Verification items for the finished model (mm, model axes). A direction names the side the tool comes from. Give positions to 0.01 mm unless a question says otherwise; leave off trailing zeros. Write each loop counter-clockwise with the first axis right and the second up, starting at its lowest first coordinate (ties: lowest second). Pieces come first, ordered by that corner, then holes. Notation, with made-up numbers: (17, 39.25) -> (49, 39.25) arc R14 cw to (49, 43.25) -> close; hole circle Ø10 at (-25.75, 89). An arc over 180 degrees is marked (long way). Answer as CSV lines item,"result".
```python
from build123d import *

# Parameters (mm, degrees)
F0_W     = 127
F0_H     = 73.025
F1_DEPTH = 22.225
F2_W     = 47.625
F2_H     = 22.225
F3_DEPTH = 6.35
F4_R     = 9.525
F5_DEPTH = 41.275


with BuildPart() as f1:
    # F0 (on Front) → F1 (new body)
    with BuildSketch(Plane.XZ):
        with Locations((0.306161, -6.260679)):
            Rectangle(F0_W, F0_H)
    extrude(amount=F1_DEPTH)

    # F2 (on face) → F3 (join)
    with BuildSketch(Plane.XY.offset(30.251821)):
        with Locations((39.993661, -11.1125)):
            Rectangle(F2_W, F2_H)
        with Locations((-39.381339, -11.1125)):
            Rectangle(F2_W, F2_H)
    extrude(amount=F3_DEPTH)

    # F4 (on face) → F5 (cut)
    with BuildSketch(Plane.XY.offset(36.601821)):
        with Locations((-34.618839, -11.1125)):
            Circle(F4_R)
        with Locations((41.581161, -11.1125)):
            Circle(F4_R)
    extrude(amount=-F5_DEPTH, mode=Mode.SUBTRACT)


solid = f1.part
```
1) Section check A-A (y = -14.5). Record the boundary of the cut face in (x, z).
Reported:
outline,"(-63.19, -42.77) -> (63.81, -42.77) -> (63.81, 36.6) -> (50.48, 36.6) -> (50.48, -4.67) -> (32.68, -4.67) -> (32.68, 36.6) -> (16.18, 36.6) -> (16.18, 30.25) -> (-15.57, 30.25) -> (-15.57, 36.6) -> (-25.72, 36.6) -> (-25.72, -4.67) -> (-43.52, -4.67) -> (-43.52, 36.6) -> (-63.19, 36.6) -> close"
2) Section check C-C (z = 0). State how many separate pieces and enclosed holes the cut face has, and give its area (3 significant figures).
Reported:
separate pieces,"1"
enclosed holes,"2"
area,"2,250 mm²"
3) Tool access check on faces 1 (the flat face through (41, -11, -4.673)), 2 (the flat face through (16.181, -11, 33)), 3 (the flat face through (-1, 0, -4)). Record the directions out of +Z, -Z, +X, -X, +Y, -Y that give a thin tool (end or side, any length) a straight path to the whole face; none if there is none.
Reported:
face 1,"+Z"
face 2,"+Z, +Y, -Y"
face 3,"+Z, -Z, +X, -X, +Y"
4) Scan lines: line 1 along X through (y, z) = (-10.5, 28.5); line 2 along X through (y, z) = (-7.5, 18.5); line 3 along Z through (x, y) = (38.5, -7.5). Record each from-to range of solid material in increasing order.
Reported:
line 1,"-63.19 to -44.12, -25.11 to 32.08, 51.09 to 63.81"
line 2,"-63.19 to -43.43, -25.81 to 32.77, 50.39 to 63.81"
line 3,"-42.77 to -4.67"
5) Section check B-B (x = -41). Record the boundary of the cut face in (y, z) (3 decimals).
Reported:
outline,"(-22.225, -42.773) -> (0, -42.773) -> (0, 36.602) -> (-4.041, 36.602) -> (-4.041, -4.673) -> (-18.184, -4.673) -> (-18.184, 36.602) -> (-22.225, 36.602) -> close"
6) Section check D-D (x = 38). Record the boundary of the cut face in (y, z) (3 decimals), and give its area (3 significant figures).
Reported:
outline,"(-22.225, -42.773) -> (0, -42.773) -> (0, 36.602) -> (-2.286, 36.602) -> (-2.286, -4.673) -> (-19.939, -4.673) -> (-19.939, 36.602) -> (-22.225, 36.602) -> close"
area,"1,040 mm²"
7) Depth check by flat-ended pin: pin 1 (11 mm diameter, centred on x = 8, y = -8, fed in from +Z); pin 2 (9.5 mm diameter, centred on x = -32, y = -8.5, fed in from +Z). Enter the tip coordinate at first touch or a pass-through.
Reported:
pin 1,"z = 30.25"
pin 2,"z = -4.67"
